Autodesk Inventor part; units mm, degrees
ref_plane "YZ Plane" through (0, 0, 0) normal (1, 0, 0) x (0, 1, 0)
ref_plane "XZ Plane" through (0, 0, 0) normal (0, 1, 0) x (-1, 0, 0)
ref_plane "XY Plane" through (0, 0, 0) normal (0, 0, 1) x (1, 0, 0)
sketch "Sketch1" plane through (0, 0, 0) normal (0, 0, 1) x (1, 0, 0)
  line L0 (0, 0) -> (1.071, 0)
  line L1 (0.5355, 0) -> (0.5355, -2.881)
  line L2 (0.5355, -2.881) -> (1.8385, -2.881)
  line L3 (1.8385, -2.881) -> (0.5355, -2.881)
  line L4 (0.5355, -2.881) -> (-0.7675, -2.881)
  arc A0 (0, 0) -> (-0.7675, -2.881) centre (20.5625, -7.0206) ccw
  arc A1 (1.8385, -2.881) -> (1.071, 0) centre (-19.4915, -7.0206) ccw
  line L5 (1.8385, -2.881) -> (2.7085, -2.881)
  line L6 (2.7085, -2.881) -> (5.3145, -2.881)
  line L7 (4.0115, -2.881) -> (4.0115, 0)
  line L8 (4.0115, 0) -> (3.476, 0)
  line L9 (4.0115, 0) -> (4.547, 0)
  arc A2 (3.476, 0) -> (2.7085, -2.881) centre (24.0385, -7.0206) ccw
  arc A3 (5.3145, -2.881) -> (4.547, 0) centre (-16.0155, -7.0206) ccw
  line L10 (5.3145, -2.881) -> (6.1845, -2.881)
  line L11 (6.1845, -2.881) -> (8.7905, -2.881)
  line L12 (7.4875, -2.881) -> (7.4875, 0)
  line L13 (7.4875, 0) -> (6.9515, 0)
  line L14 (7.4875, 0) -> (8.0235, 0)
  arc A4 (6.9515, 0) -> (6.1845, -2.881) centre (27.5152, -7.0172) ccw
  arc A5 (8.7905, -2.881) -> (8.0235, 0) centre (-12.5402, -7.0172) ccw
  line L15 (8.7905, -2.881) -> (9.6605, -2.881)
  line L16 (9.6605, -2.881) -> (12.2665, -2.881)
  line L17 (10.9635, -2.881) -> (10.9635, 0)
  line L18 (10.9635, 0) -> (10.4275, 0)
  line L19 (10.9635, 0) -> (11.4995, 0)
  arc A6 (10.4275, 0) -> (9.6605, -2.881) centre (30.9912, -7.0172) ccw
  arc A7 (12.2665, -2.881) -> (11.4995, 0) centre (-9.0642, -7.0172) ccw
  line L20 (-0.7675, -2.881) -> (-0.7675, -7.881)
  line L21 (12.2665, -2.881) -> (13.1365, -2.881)
  line L22 (13.1365, -2.881) -> (15.7425, -2.881)
  line L23 (14.4395, -2.881) -> (14.4395, 0)
  line L24 (14.4395, 0) -> (13.9035, 0)
  line L25 (14.4395, 0) -> (14.9755, 0)
  arc A8 (13.9035, 0) -> (13.1365, -2.881) centre (34.4672, -7.0172) ccw
  arc A9 (15.7425, -2.881) -> (14.9755, 0) centre (-5.5882, -7.0172) ccw
  line L26 (15.7425, -2.881) -> (16.6125, -2.881)
  line L27 (16.6125, -2.881) -> (19.2185, -2.881)
  line L28 (17.9155, -2.881) -> (17.9155, 0)
  line L29 (17.9155, 0) -> (17.3795, 0)
  line L30 (17.9155, 0) -> (18.4515, 0)
  arc A10 (17.3795, 0) -> (16.6125, -2.881) centre (37.9432, -7.0172) ccw
  arc A11 (19.2185, -2.881) -> (18.4515, 0) centre (-2.1122, -7.0172) ccw
  line L31 (19.2185, -2.881) -> (20.0885, -2.881)
  line L32 (20.0885, -2.881) -> (22.6945, -2.881)
  line L33 (21.3915, -2.881) -> (21.3915, 0)
  line L34 (21.3915, 0) -> (20.8555, 0)
  line L35 (21.3915, 0) -> (21.9275, 0)
  arc A12 (20.8555, 0) -> (20.0885, -2.881) centre (41.4192, -7.0172) ccw
  arc A13 (22.6945, -2.881) -> (21.9275, 0) centre (1.3638, -7.0172) ccw
  line L36 (22.6945, -2.881) -> (23.5645, -2.881)
  line L37 (23.5645, -2.881) -> (26.1705, -2.881)
  line L38 (24.8675, -2.881) -> (24.8675, 0)
  line L39 (24.8675, 0) -> (24.3315, 0)
  line L40 (24.8675, 0) -> (25.4035, 0)
  arc A14 (24.3315, 0) -> (23.5645, -2.881) centre (44.8952, -7.0172) ccw
  arc A15 (26.1705, -2.881) -> (25.4035, 0) centre (4.8398, -7.0172) ccw
  line L41 (26.1705, -2.881) -> (27.0405, -2.881)
  line L42 (27.0405, -2.881) -> (29.6465, -2.881)
  line L43 (29.6465, -2.881) -> (30.5165, -2.881)
  line L44 (30.5165, -2.881) -> (33.1225, -2.881)
  line L45 (33.1225, -2.881) -> (33.9925, -2.881)
  line L46 (33.9925, -2.881) -> (36.5985, -2.881)
  line L47 (36.5985, -2.881) -> (37.4685, -2.881)
  line L48 (37.4685, -2.881) -> (40.0745, -2.881)
  line L49 (40.0745, -2.881) -> (40.9445, -2.881)
  line L50 (40.9445, -2.881) -> (43.5505, -2.881)
  line L51 (43.5505, -2.881) -> (44.4205, -2.881)
  line L52 (44.4205, -2.881) -> (47.0265, -2.881)
  line L53 (47.0265, -2.881) -> (47.8965, -2.881)
  line L54 (47.8965, -2.881) -> (50.5025, -2.881)
  line L55 (50.5025, -2.881) -> (51.3725, -2.881)
  line L56 (51.3725, -2.881) -> (53.9785, -2.881)
  line L57 (53.9785, -2.881) -> (53.9785, -7.881)
  line L58 (53.9785, -7.881) -> (-0.7675, -7.881)
  line L59 (28.3435, -2.881) -> (28.3435, 0)
  line L60 (31.8195, -2.881) -> (31.8195, 0)
  line L61 (31.8195, 0) -> (31.2835, 0)
  line L62 (35.2955, -2.881) -> (35.2955, 0)
  line L63 (35.2955, 0) -> (34.7595, 0)
  line L64 (38.7715, -2.881) -> (38.7715, 0)
  line L65 (38.7715, 0) -> (38.2355, 0)
  line L66 (42.2475, -2.881) -> (42.2475, 0)
  line L67 (42.2475, 0) -> (41.7115, 0)
  line L68 (45.7235, -2.881) -> (45.7235, 0)
  line L69 (45.7235, 0) -> (45.1875, 0)
  line L70 (49.1995, -2.881) -> (49.1995, 0)
  line L71 (49.1995, 0) -> (48.6635, 0)
  line L72 (52.6755, -2.881) -> (52.6755, 0)
  line L73 (52.6755, 0) -> (52.1395, 0)
  line L74 (52.6755, 0) -> (53.2115, 0)
  line L75 (49.1995, 0) -> (49.7355, 0)
  line L76 (45.7235, 0) -> (46.2595, 0)
  line L77 (42.2475, 0) -> (42.7835, 0)
  line L78 (38.7715, 0) -> (39.3075, 0)
  line L79 (35.2955, 0) -> (35.8315, 0)
  line L80 (31.8195, 0) -> (32.3555, 0)
  line L81 (28.3435, 0) -> (28.8795, 0)
  line L82 (28.3435, 0) -> (27.8075, 0)
  arc A16 (27.8075, 0) -> (27.0405, -2.881) centre (48.3712, -7.0172) ccw
  arc A17 (29.6465, -2.881) -> (28.8795, 0) centre (8.3158, -7.0172) ccw
  arc A18 (31.2835, 0) -> (30.5165, -2.881) centre (51.8472, -7.0172) ccw
  arc A19 (33.1225, -2.881) -> (32.3555, 0) centre (11.7918, -7.0172) ccw
  arc A20 (34.7595, 0) -> (33.9925, -2.881) centre (55.3232, -7.0172) ccw
  arc A21 (36.5985, -2.881) -> (35.8315, 0) centre (15.2678, -7.0172) ccw
  arc A22 (38.2355, 0) -> (37.4685, -2.881) centre (58.7992, -7.0172) ccw
  arc A23 (40.0745, -2.881) -> (39.3075, 0) centre (18.7438, -7.0172) ccw
  arc A24 (41.7115, 0) -> (40.9445, -2.881) centre (62.2752, -7.0172) ccw
  arc A25 (43.5505, -2.881) -> (42.7835, 0) centre (22.2198, -7.0172) ccw
  arc A26 (45.1875, 0) -> (44.4205, -2.881) centre (65.7512, -7.0172) ccw
  arc A27 (47.0265, -2.881) -> (46.2595, 0) centre (25.6958, -7.0172) ccw
  arc A28 (48.6635, 0) -> (47.8965, -2.881) centre (69.2272, -7.0172) ccw
  arc A29 (50.5025, -2.881) -> (49.7355, 0) centre (29.1718, -7.0172) ccw
  arc A30 (52.1395, 0) -> (51.3725, -2.881) centre (72.7032, -7.0172) ccw
  arc A31 (53.9785, -2.881) -> (53.2115, 0) centre (32.6478, -7.0172) ccw
  dimension "d0" = 1.071
  dimension "d1" = 2.881
  dimension "d3" = 1.303
  dimension "d4" = 1.303
  dimension "d5" = 21.728
  dimension "d6" = 21.728
  dimension "d7" = 0.87
  dimension "d8" = 2.606
  dimension "d9" = 0.5355
  dimension "d10" = 0.5355
  dimension "d11" = 21.728
  dimension "d12" = 21.728
  dimension "d13" = 0.87
  dimension "d14" = 2.606
  dimension "d15" = 0.536
  dimension "d16" = 0.536
  dimension "d17" = 21.728
  dimension "d18" = 21.728
  dimension "d19" = 0.87
  dimension "d20" = 2.606
  dimension "d21" = 0.536
  dimension "d22" = 0.536
  dimension "d23" = 21.728
  dimension "d24" = 21.728
  dimension "d25" = 5
  dimension "d27" = 0.87
  dimension "d28" = 2.606
  dimension "d29" = 0.536
  dimension "d30" = 0.536
  dimension "d31" = 21.728
  dimension "d32" = 21.728
  dimension "d33" = 0.87
  dimension "d34" = 2.606
  dimension "d35" = 0.536
  dimension "d36" = 0.536
  dimension "d37" = 21.728
  dimension "d38" = 21.728
  dimension "d39" = 0.87
  dimension "d40" = 2.606
  dimension "d41" = 0.536
  dimension "d42" = 0.536
  dimension "d43" = 21.728
  dimension "d44" = 21.728
  dimension "d45" = 0.87
  dimension "d46" = 2.606
  dimension "d47" = 0.536
  dimension "d48" = 0.536
  dimension "d49" = 21.728
  dimension "d50" = 21.728
  dimension "d51" = 0.87
  dimension "d52" = 2.606
  dimension "d53" = 0.87
  dimension "d54" = 2.606
  dimension "d55" = 0.87
  dimension "d56" = 2.606
  dimension "d57" = 0.87
  dimension "d58" = 2.606
  dimension "d59" = 0.87
  dimension "d60" = 2.606
  dimension "d61" = 0.87
  dimension "d62" = 2.606
  dimension "d63" = 0.87
  dimension "d64" = 2.606
  dimension "d65" = 0.87
extrude "Extrusion1" add sketch "Sketch1" along normal blind 10
sketch "Sketch3" plane through (-0.7675, -7.881, 0) normal (0, -1, 0) x (1, 0, 0)
  circle A0 centre (27.373, 5) radius 3.5
  line L0 (54.746, 0) -> (54.746, 10)
  line L1 (0, 0) -> (54.746, 0)
  point P0 (0.7675, 0)
  dimension "d104" = 7
  dimension "d105" = 27.373
  dimension "d106" = 5
extrude "Extrusion3" cut sketch "Sketch3" against normal blind 3
properties part number "1p10 DP3 gear attachment"
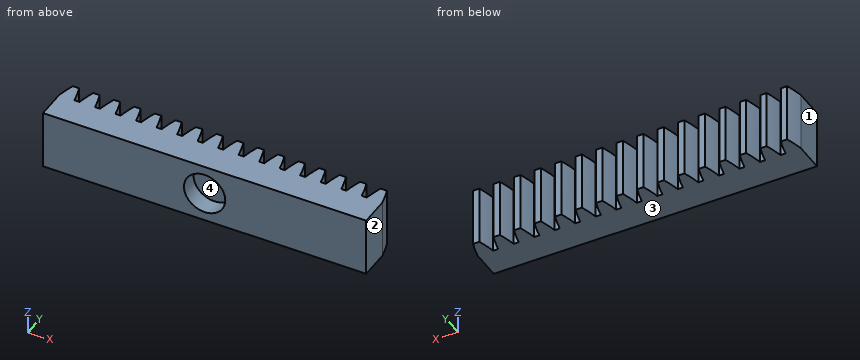
Model file for the job. Use its own axes, mm. Face numbers are marked on the shaded views. Coordinates: 2 decimals unless noted, no trailing zeros. Order: outer loops, then holes, each group sorted by start corner. A loop starts at its lowest first (then second) coordinate and runs counter-clockwise, first axis right, second up. Notation, with made-up numbers: (51, 56.25) - (73, 56.25) arc R22 cw to (73, 89.25) - close; hole circle Ø8 at (21.25, 12.5). An arc over 180 degrees is marked (long way). Return JSON: item names as keys, results as strings. Group by question number.
1) Probe line 1 (Y direction, x = 23.5, z = 0.5); line 2 (Y direction, x = 26.5, z = 8.25). List the from-to ranges inside material, lowest first. Write a range as from..to.
2) Mould opens along X. For the marked faces 1, 2, 3 and 4 say: released by +X, released by -X, zero draft, split by the parting line, or undercut.
3) Saw through at A-A, the plane y = -6. Write the cut outline in (x, z).
4) Flat gauge pin, fed straight in: P1, Ø2, axis at x = 28, z = 5, coming from the -Y side. Where does the tip first touch, or does it go through?
5) Saw through at B-B, the plane y = -1.75. Count the separate pieces of the cut face and the enclosed holes in it, plus the area to 3 significant figures.
Values found:
{
 "1": {"line 1": "y = -7.88..-2.88", "line 2": "y = -4.88..-2.88"},
 "2": {"face 1": "released by -X", "face 2": "released by +X", "face 3": "zero draft", "face 4": "undercut"},
 "3": {"outline": "(-0.77, 0) - (53.98, 0) - (53.98, 10) - (-0.77, 10) - close; hole circle Ø7 at (26.61, 5)"},
 "4": {"P1": "stops at y = -4.88"},
 "5": {"separate pieces": "16", "enclosed holes": "0", "area": "337 mm²"}
}
